Read the model definition and answer for the solid it produces. Units are mm, in the model's axes. Face numbers are marked on the shaded views. A direction names the side the tool comes from. Coordinates: 2 decimals unless noted, no trailing zeros. Order: outer loops, then holes, each group sorted by start corner. A loop starts at its lowest first (then second) coordinate and runs counter-clockwise, first axis right, second up. Notation, with made-up numbers: (38, -25) -> (68, -25) arc R18 cw to (68, 5) -> close; hole circle Ø11 at (-2, 31). An arc over 180 degrees is marked (long way). Use CSV: the item, a comma, the result in double quotes.
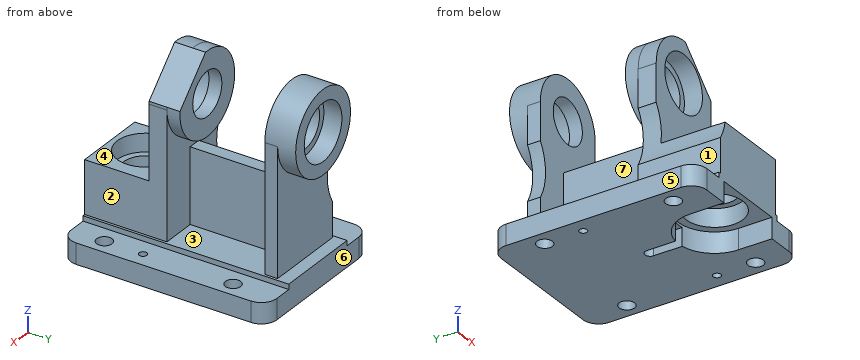
```python
from build123d import *

# Parameters (mm, degrees)
EXTRUDE_1_DEPTH           = 8
SKETCH_3_W                = 34
SKETCH_3_H                = 80
EXTRUDE_2_DEPTH           = 2
CUT_EXTRUDE_1_DEPTH       = 8
CUT_EXTRUDE_2_DEPTH       = 7
SKETCH_6_W                = 32
SKETCH_6_H                = 25
EXTRUDE_4_DEPTH           = 20.5
SKETCH_7_R                = 11
CUT_EXTRUDE_5_DEPTH       = 7
SKETCH_8_R                = 8.5
CUT_EXTRUDE_6_DEPTH       = 8.5
SKETCH_9_R                = 11
CUT_EXTRUDE_7_DEPTH       = 7
EXTRUDE_5_DEPTH           = 7
EXTRUDE_6_DEPTH           = 5
SKETCH_13_R               = 8.5
CUT_EXTRUDE_8_DEPTH       = 5
SKETCH_14_R               = 11
CUT_EXTRUDE_9_DEPTH       = 7
SKETCH_15_R               = 8.5
EXTRUDE_7_DEPTH           = 5
SKETCH_16_R               = 16
SKETCH_16_R_2             = 11
EXTRUDE_8_DEPTH           = 7
F_6_0MM_START             = -8
F_6_0MM_1_OUTLINE_R       = 3
F_6_0MM_1_DEPTH           = 8
F_3_0MM_1_D               = 3
RIB_13_REACH              = 86.734
SKETCH_21_WALL_W          = 209.467873062
SKETCH_21_WALL_H          = 5
CUT_EXTRUDE_10_DEPTH      = 102.56692375
CUT_EXTRUDE_10_DEPTH_BACK = 102.56692375
SKETCH_23_R               = 20


# Read off the part's stored shape, not the designer's step: Ø6.0mm 暗销孔1
with BuildPart() as part:
    # 草图1 → 凸台-拉伸1 (new body)
    with BuildSketch(Plane.XY):
        with BuildLine():
            Line((24, -40), (-24, -40))
            ThreePointArc((-24, -40), (-28.242640687, -38.242640687), (-30, -34))
            Line((-30, -34), (-30, 34))
            ThreePointArc((-30, 34), (-28.242640687, 38.242640687), (-24, 40))
            Line((-24, 40), (24, 40))
            ThreePointArc((24, 40), (28.242640687, 38.242640687), (30, 34))
            Line((30, 34), (30, -34))
            ThreePointArc((30, -34), (28.242640687, -38.242640687), (24, -40))
        make_face()
    extrude(amount=-EXTRUDE_1_DEPTH)

    # 草图3 → 凸台-拉伸2 (add)
    with BuildSketch(Plane.XY):
        Rectangle(SKETCH_3_W, SKETCH_3_H)
    extrude(amount=EXTRUDE_2_DEPTH)

    # 草图4 → 切除-拉伸1 (cut)
    with BuildSketch(Plane(origin=(0, 0, -8), x_dir=(-1, 0, 0), z_dir=(0, 0, -1))):
        with BuildLine():
            Line((-14, -27), (-14, -40))
            Line((-14, -40), (14, -40))
            Line((14, -40), (14, -27))
            ThreePointArc((14, -27), (0, -13), (-14, -27))
        make_face()
    extrude(amount=-CUT_EXTRUDE_1_DEPTH, mode=Mode.SUBTRACT)

    # 草图5 → 切除-拉伸2 (cut)
    with BuildSketch(Plane(origin=(0, 0, -8), x_dir=(-1, 0, 0), z_dir=(0, 0, -1))):
        with BuildLine():
            Line((-2, -2), (-2, -13.143593539))
            ThreePointArc((-2, -13.143593539), (0, -13), (2, -13.143593539))
            Line((2, -13.143593539), (2, -2))
            ThreePointArc((2, -2), (0, 0), (-2, -2))
        make_face()
    extrude(amount=-CUT_EXTRUDE_2_DEPTH, mode=Mode.SUBTRACT)

    # 草图6 → 凸台-拉伸4 (add)
    with BuildSketch(Plane.XY.offset(2)):
        with Locations((0, -27.5)):
            Rectangle(SKETCH_6_W, SKETCH_6_H)
    extrude(amount=EXTRUDE_4_DEPTH)

    # 草图7 → 切除-拉伸5 (cut)
    with BuildSketch(Plane(origin=(0, 0, 0), x_dir=(-1, 0, 0), z_dir=(0, 0, -1))):
        with Locations((0, -27)):
            Circle(SKETCH_7_R)
    extrude(amount=-CUT_EXTRUDE_5_DEPTH, mode=Mode.SUBTRACT)

    # 草图8 → 切除-拉伸6 (cut)
    with BuildSketch(Plane(origin=(0, 0, 7), x_dir=(-1, 0, 0), z_dir=(0, 0, -1))):
        with Locations((0, -27)):
            Circle(SKETCH_8_R)
    extrude(amount=-CUT_EXTRUDE_6_DEPTH, mode=Mode.SUBTRACT)

    # 草图9 → 切除-拉伸7 (cut)
    with BuildSketch(Plane(origin=(0, 0, 15.5), x_dir=(-1, 0, 0), z_dir=(0, 0, -1))):
        with Locations((0, -27)):
            Circle(SKETCH_9_R)
    extrude(amount=-CUT_EXTRUDE_7_DEPTH, mode=Mode.SUBTRACT)

    # 草图11 → 凸台-拉伸5 (add)
    with BuildSketch(Plane(origin=(0, -15, 0), x_dir=(1, 0, 0), z_dir=(0, 1, 0))):
        with BuildLine():
            Line((-16, -2), (16, -2))
            Line((16, -2), (16, -51.2))
            ThreePointArc((16, -51.2), (15.99214711, -51.701229307), (15.968596148, -52.201966601))
            Line((15.968596148, -52.201966601), (1.001966601, -67.168596148))
            ThreePointArc((1.001966601, -67.168596148), (-10.953733026, -62.862578309), (-16, -51.2))
            Line((-16, -51.2), (-16, -2))
        make_face()
    extrude(amount=EXTRUDE_5_DEPTH)

    # 草图12 → 凸台-拉伸6 (add)
    with BuildSketch(Plane(origin=(0, -8, 0), x_dir=(1, 0, 0), z_dir=(0, 1, 0))):
        with BuildLine():
            Line((1.001966601, -67.168596148), (15.968596148, -52.201966601))
            ThreePointArc((15.968596148, -52.201966601), (-11.313708499, -39.886291501), (1.001966601, -67.168596148))
        make_face()
    extrude(amount=EXTRUDE_6_DEPTH)

    # 草图13 → 切除-拉伸8 (cut)
    with BuildSketch(Plane(origin=(0, -3, 0), x_dir=(1, 0, 0), z_dir=(0, 1, 0))):
        with Locations(Location((0, -51.2, 0), (0, 0, 270))):
            Circle(SKETCH_13_R)
    extrude(amount=-CUT_EXTRUDE_8_DEPTH, mode=Mode.SUBTRACT)

    # 草图14 → 切除-拉伸9 (cut)
    with BuildSketch(Plane(origin=(0, -8, 0), x_dir=(1, 0, 0), z_dir=(0, 1, 0))):
        with Locations(Location((0, -51.2, 0), (0, 0, 270))):
            Circle(SKETCH_14_R)
    extrude(amount=-CUT_EXTRUDE_9_DEPTH, mode=Mode.SUBTRACT)

    # 草图15 → 凸台-拉伸7 (add)
    with BuildSketch(Plane(origin=(0, 30, 0), x_dir=(1, 0, 0), z_dir=(0, 1, 0))):
        with BuildLine():
            Line((-16, -2), (16, -2))
            Line((16, -2), (16, -51.2))
            ThreePointArc((16, -51.2), (0, -67.2), (-16, -51.2))
            Line((-16, -51.2), (-16, -2))
        make_face()
        with Locations(Location((0, -51.2, 0), (0, 0, 270))):
            Circle(SKETCH_15_R, mode=Mode.SUBTRACT)
    extrude(amount=EXTRUDE_7_DEPTH)

    # 草图16 → 凸台-拉伸8 (add)
    with BuildSketch(Plane(origin=(0, 35, 0), x_dir=(1, 0, 0), z_dir=(0, 1, 0))):
        with Locations((0, -51.2)):
            Circle(SKETCH_16_R)
        with Locations(Location((0, -51.2, 0), (0, 0, 270))):
            Circle(SKETCH_16_R_2, mode=Mode.SUBTRACT)
    extrude(amount=EXTRUDE_8_DEPTH)

    # Ø6.0mm 暗销孔1 outline → Ø6.0mm 暗销孔1 (cut)
    with BuildSketch(Plane.XY.offset(F_6_0MM_START)):
        with Locations((-24, -27)):
            Circle(F_6_0MM_1_OUTLINE_R)
        with Locations((24, 23)):
            Circle(F_6_0MM_1_OUTLINE_R)
        with Locations((24, -27)):
            Circle(F_6_0MM_1_OUTLINE_R)
        with Locations((-24, 23)):
            Circle(F_6_0MM_1_OUTLINE_R)
    extrude(amount=F_6_0MM_1_DEPTH, mode=Mode.SUBTRACT)

    # Ø3.0mm 暗销孔1 (through all)
    with Locations(Plane.XY):
        with Locations((24, -12), (-24, 8)):
            Hole(F_3_0MM_1_D / 2)

    # 草图21 wall → 筋13 (add, up to next)
    with BuildSketch(Plane(origin=(0, 11, 31), x_dir=(0, -1, 0), z_dir=(0, 0, -1)), mode=Mode.PRIVATE) as rib_13_sk1:
        Rectangle(SKETCH_21_WALL_W, SKETCH_21_WALL_H)
    rib_13_tool1 = extrude(rib_13_sk1.sketch, amount=RIB_13_REACH, mode=Mode.PRIVATE) - part.part
    add(rib_13_tool1.solids().sort_by_distance((0, 11, 31))[0])

    # 草图23 → 切除-拉伸10 (cut, two sides: drawn at the far end of the back side and taken through both)
    with BuildSketch(Plane(origin=(0, 30, 0), x_dir=(1, 0, 0), z_dir=(0, 1, 0)).offset(-CUT_EXTRUDE_10_DEPTH_BACK)):
        with Locations((-33, -26)):
            Circle(SKETCH_23_R)
    extrude(amount=CUT_EXTRUDE_10_DEPTH + CUT_EXTRUDE_10_DEPTH_BACK, mode=Mode.SUBTRACT)


solid = part.part
```
Item 1: Find section A-A, the plane y = 23. Give the vertices of the cut face in (x, z).
Return value:
outline,"(-30, -8) -> (-27, -8) -> (-27, 0) -> (-30, 0) -> close; (-21, -8) -> (21, -8) -> (21, 0) -> (17, 0) -> (17, 2) -> (2.5, 2) -> (2.5, 31) -> (-2.5, 31) -> (-2.5, 2) -> (-17, 2) -> (-17, 0) -> (-21, 0) -> close; (27, -8) -> (30, -8) -> (30, 0) -> (27, 0) -> close"
Item 2: Each of these flat-tipped pins is pushed along its axis until it touches: P1, Ø2.5, axis at y = 33, z = 7, coming from the -X side; P2, Ø3.5, axis at x = 24, y = -12, coming from the +Z side; P3, Ø1.5, axis at x = 16, z = 9.5, coming from the +Y side; P4, Ø1.6, axis at y = 7.5, z = 0.5, coming from the -X side. Where does it stop, or does it pass through?
Return value:
P1,"stops at x = -16"
P2,"stops at z = 0"
P3,"stops at y = 35"
P4,"stops at x = -30"
Item 3: Find section B-B, the plane z = 14. Give the vertices of the cut face in (x, y), then the cut area to 3 significant figures.
Return value:
outline,"(-16, -40) -> (16, -40) -> (16, -8) -> (2.5, -8) -> (2.5, 30) -> (16, 30) -> (16, 35) -> (-16, 35) -> (-16, 30) -> (-2.5, 30) -> (-2.5, -8) -> (-16, -8) -> close; hole circle Ø17 at (0, -27)"
area,"1,150 mm^2"
Item 4: A tool of negligible diameter and unlimited length cuts with its end or side. For the marked faces 1, 2, 3 and 4, from which of +Z, -Z, +X, -X, +Y, -Y can it reach the whole face along a straight path? Write none if from no direction.
Return value:
face 1,"+Z, -X, +Y, -Y"
face 2,"+Z, +X, +Y, -Y"
face 3,"none"
face 4,"+Z, +X, -X, -Y"
Item 5: Straight lines are drawn through the part: line 1 along Y through (x, z) = (-24, -1.75); line 2 along Y through (x, z) = (24, -5); line 3 along Y through (x, z) = (-10.5, 60). For each, find the intervals that lie inside material, in ascending order.
Return value:
line 1,"y = -40 to -30, -24 to 6.5, 9.5 to 20, 26 to 40"
line 2,"y = -40 to -30, -24 to -13.5, -10.5 to 20, 26 to 40"
line 3,"y = -15 to -3, 30 to 42"
Item 6: Find section C-C, the plane y = 8. Give the vertices of the cut face in (x, z), then the cut area to 3 significant figures.
Return value:
outline,"(-30, -8) -> (-25.5, -8) -> (-25.5, 0) -> (-30, 0) -> close; (-22.5, -8) -> (30, -8) -> (30, 0) -> (17, 0) -> (17, 2) -> (2.5, 2) -> (2.5, 31) -> (-2.5, 31) -> (-2.5, 2) -> (-17, 2) -> (-17, 0) -> (-22.5, 0) -> close"
area,"669 mm^2"
Item 7: Find section D-D, the plane z = 56.5. Give the vertices of the cut face in (x, y).
Return value:
outline,"(-15.1, -15) -> (-9.64, -15) -> (-9.64, -8) -> (-6.65, -8) -> (-6.65, -3) -> (-15.1, -3) -> close; (-15.1, 30) -> (-6.65, 30) -> (-6.65, 35) -> (-9.64, 35) -> (-9.64, 42) -> (-15.1, 42) -> close; (6.65, -8) -> (9.64, -8) -> (9.64, -15) -> (11.67, -15) -> (11.67, -3) -> (6.65, -3) -> close; (6.65, 30) -> (15.1, 30) -> (15.1, 42) -> (9.64, 42) -> (9.64, 35) -> (6.65, 35) -> close"
Item 8: The mould has two halves that part along Y. Classify the marked faces 5, 6 and 7: +Y half, -Y half, draft (parallel to the pull), parting line (faces both ways), or undercut.
Return value:
face 5,"draft"
face 6,"+Y half"
face 7,"undercut"
